```python
from build123d import *

# Parameters (mm, degrees)
EXTRUDE_1_DEPTH             = 3
EXTRUDE_2_DEPTH             = 3
CUT_EXTRUDE_1_DEPTH         = 1
CUT_EXTRUDE_2_DEPTH         = 1
HOLE_WIZARD_3_4_3_4_1_D     = 3.4
HOLE_WIZARD_3_4_3_4_1_DEPTH = 55
FILLET_1_R                  = 3


with BuildPart() as part:
    # 草图1 → 凸台-拉伸1 (new body)
    with BuildSketch(Plane(origin=(0, 177.5, 0), x_dir=(1, 0, 0), z_dir=(0, 1, 0))):
        Polygon((920, -15), (925, -3), (875, -3), (880, -15), align=None)
    extrude(amount=-EXTRUDE_1_DEPTH)

    # 草图2 → 凸台-拉伸2 (add)
    with BuildSketch(Plane(origin=(0, 0, 3), x_dir=(-1, 0, 0), z_dir=(0, 0, -1))):
        with BuildLine():
            Line((-925, 147.5), (-925, 177.5))
            Line((-925, 177.5), (-875, 177.5))
            Line((-875, 177.5), (-875, 147.5))
            ThreePointArc((-875, 147.5), (-900, 122.5), (-925, 147.5))
        make_face()
    extrude(amount=EXTRUDE_2_DEPTH)

    # 草图3 → 切除-拉伸1 (cut)
    with BuildSketch(Plane.XZ.offset(-174.5)):
        Polygon((912.142116168, 12.65), (912.142116168, 9.35), (915, 7.7), (917.857883832, 9.35), (917.857883832, 12.65), (915, 14.3), align=None)
    extrude(amount=-CUT_EXTRUDE_1_DEPTH, mode=Mode.SUBTRACT)

    # 草图4 → 切除-拉伸2 (cut)
    with BuildSketch(Plane.XZ.offset(-174.5)):
        Polygon((882.142116168, 9.35), (885, 7.7), (887.857883832, 9.35), (887.857883832, 12.65), (885, 14.3), (882.142116168, 12.65), align=None)
    extrude(amount=-CUT_EXTRUDE_2_DEPTH, mode=Mode.SUBTRACT)

    # Ø3.4 (3.4) 直径孔1
    with Locations(Plane(origin=(0, 177.5, 0), x_dir=(1, 0, 0), z_dir=(0, 1, 0))):
        with Locations((885, -11), (915, -11)):
            Hole(HOLE_WIZARD_3_4_3_4_1_D / 2, depth=HOLE_WIZARD_3_4_3_4_1_DEPTH)

    # 圆角1
    fillet_1_edges = [part.edges().sort_by_distance(p)[0] for p in [
        (900, 174.5, 3),
        (880, 176, 15),
        (920, 176, 15),
    ]]
    fillet(fillet_1_edges, radius=FILLET_1_R)


solid = part.part
```
Can you work these out from the model? Positions are in its coordinate system, mm. A direction names the side the tool comes from. Give positions to 0.01 mm unless a question says otherwise; leave off trailing zeros. Order: outer loops, then holes, each group sorted by start corner. A loop starts at its lowest first (then second) coordinate and runs counter-clockwise, first axis right, second up. Notation, with made-up numbers: (68.25, 58) - (112.25, 58) arc R25 ccw to (112.25, 86) - close; hole circle Ø5 at (61.25, 20.5). An arc over 180 degrees is marked (long way). Use a Markdown table: item, result. Add a question column.
Q1. If we mould it in two halves opening along X, with no side actions, what happens to faces 4 (the cylindrical face through (899.65, 173.6, 3.86)), 5 (the flat face through (877.086, 175.875, 8.006)), 6 (the flat face through (913.551, 174.993, 8.537)), 7 (the flat face through (925, 162, 2))? For each: released by +X, released by -X, zero draft, split by the parting line, or undercut.
Q2. On a 3-axis mill with a long thin cutter (end or side, diameter ignored), from which of +Z, -Z, +X, -X, +Y, -Y can I reach the whole of each face in a straight line? I mean faces 1 (the flat face through (900, 147, 3)), 2 (the flat face through (922.855, 175.875, 8.148)), 3 (the flat face through (916.23, 175.5, 9.58)). Say none if no direction works.
Q3. I'm going to push flat-ended pins straight in: pin 1 (4.5 mm diameter, centred on x = 885, z = 11, fed in from -Y); pin 2 (1.5 mm diameter, centred on x = 904.5, z = 7, fed in from -Y); pin 3 (1.1 mm diameter, centred on y = 175, z = 11.5, fed in from -X). Where does each tip first touch, or does it pass through?
Q4. If we section it at A-A on x = 900: Write out the boundary of the cut face in (y, z).
Q5. Please list where these lines run through material, in increasing order: line 1 along Z through (x, y) = (885, 176.3); line 2 along X through (y, z) = (177, 11); line 3 along Z through (x, y) = (914, 168).
Q6. If we section it at B-B on z = 11: Write out the boundary of the cut face in (x, y).
Q7. If we section it at D-D on y = 143.5: Write out the boundary of the cut face in (x, z), plus the area to 3 significant figures.
Q8. If we section it at C-C on z = 1.25: Write out the boundary of the cut face in (x, y).
Answers follow:
| question | item | result |
|---|---|---|
| 1 | face 4 | zero draft |
| 1 | face 5 | released by -X |
| 1 | face 6 | undercut |
| 1 | face 7 | released by +X |
| 2 | face 1 | +Z, +X, -X, -Y |
| 2 | face 2 | +Z, +X, +Y, -Y |
| 2 | face 3 | -Y |
| 3 | pin 1 | stops at y = 175.5 |
| 3 | pin 2 | stops at y = 174.5 |
| 3 | pin 3 | stops at x = 878.31 |
| 4 | outline | (122.5, 0) - (177.5, 0) - (177.5, 15) - (174.5, 15) - (174.5, 6) arc R3 cw to (171.5, 3) - (122.5, 3) - close |
| 5 | line 1 | z = 0 to 9.3, 12.7 to 15 |
| 5 | line 2 | x = 878.33 to 883.3, 886.7 to 913.3, 916.7 to 921.67 |
| 5 | line 3 | z = 0 to 3 |
| 6 | outline | (878.33, 174.5) - (882.14, 174.5) - (882.14, 175.5) - (883.3, 175.5) - (883.3, 177.5) - (878.33, 177.5) - close; (886.7, 175.5) - (887.86, 175.5) - (887.86, 174.5) - (912.14, 174.5) - (912.14, 175.5) - (913.3, 175.5) - (913.3, 177.5) - (886.7, 177.5) - close; (916.7, 175.5) - (917.86, 175.5) - (917.86, 174.5) - (921.67, 174.5) - (921.67, 177.5) - (916.7, 177.5) - close |
| 7 | outline | (875.32, 0) - (924.68, 0) - (924.68, 3) - (875.32, 3) - close |
| 7 | area | 148 mm^2 |
| 8 | outline | (875, 147.5) arc R25 ccw to (925, 147.5) - (925, 177.5) - (875, 177.5) - close |
